Read the model definition and answer for the solid it produces. Units are mm, in the model's axes. A direction names the side the tool comes from. Give positions to 0.01 mm unless a question says otherwise; leave off trailing zeros. Order: outer loops, then holes, each group sorted by start corner. A loop starts at its lowest first (then second) coordinate and runs counter-clockwise, first axis right, second up. Notation, with made-up numbers: (49.25, -23.75) - (58.25, -23.75) arc R20 ccw to (58.25, -8.75) - close; hole circle Ø5 at (19, 63.25). An arc over 180 degrees is marked (long way). Write item = value, one per line.
```python
from build123d import *

# Parameters (mm, degrees)
F1_DEPTH = 5


with BuildPart() as f1:
    # F0 (on Front) → F1 (new body)
    with BuildSketch(Plane.XZ):
        Polygon((61.512955, -18.03444), (75.960928, 2.436688), (64.075245, 1.856776), (71.490157, 25.790645), (60.365404, 21.566239), (60.021432, 46.620035), (50.746576, 39.164648), (42.677391, 62.885931), (36.16032, 52.929348), (21.15579, 72.996113), (18.03444, 61.512955), (-2.436688, 75.960928), (-1.856776, 64.075245), (-25.790645, 71.490157), (-21.566239, 60.365404), (-46.620035, 60.021432), (-39.164648, 50.746576), (-62.885931, 42.677391), (-52.929348, 36.16032), (-72.996113, 21.15579), (-61.512955, 18.03444), (-75.960928, -2.436688), (-64.075245, -1.856776), (-71.490157, -25.790645), (-60.365404, -21.566239), (-60.021432, -46.620035), (-50.746576, -39.164648), (-42.677391, -62.885931), (-36.16032, -52.929348), (-21.15579, -72.996113), (-18.03444, -61.512955), (2.436688, -75.960928), (1.856776, -64.075245), (25.790645, -71.490157), (21.566239, -60.365404), (46.620035, -60.021432), (39.164648, -50.746576), (62.885931, -42.677391), (52.929348, -36.16032), (72.996113, -21.15579), align=None)
        with BuildLine():
            ThreePointArc((3.847568, 18.606349), (14.732681, 11.997837), (19, 0))
            ThreePointArc((19, 0), (-12.106443, -14.643566), (-3.572003, 18.661211))
            Line((-3.572003, 18.661211), (-3.572003, 23.642808))
            Line((-3.572003, 23.642808), (3.847568, 23.642808))
            Line((3.847568, 23.642808), (3.847568, 18.606349))
        make_face(mode=Mode.SUBTRACT)
    extrude(amount=F1_DEPTH)


solid = f1.part
```
1. Straight lines are drawn through the part: L1, parallel to Z at x = 56, y = -1.5; L2, parallel to Z at x = 16, y = -3.4; L3, parallel to X at y = -4.2, z = 5. For each, find the intervals that lie inside material, in ascending order. Write a range as [from, to].
Recorded:
L1 = [-45.02, -38.17], [-33.86, 43.39]
L2 = [-68.46, -10.25], [10.25, 62.95]
L3 = [-70.71, -18.33], [18.33, 65.05]
2. Flat-ended cylindrical pins translate along their axes: pin 1 (1 mm diameter, centred on x = 36.5, y = -4.5, fed in from +Z); pin 2 (2 mm diameter, centred on y = -3.5, z = -53.5, fed in from +X). Find the tip coordinate at first contact, or state that the pin passes through.
Recorded:
pin_1 = 54.21
pin_2 = 42.18
3. Section D-D (z = -30.5) is taken. Determine the outline of the cut face in (x, y).
Recorded:
outline = (-60.24, -5) - (60.5, -5) - (60.5, 0) - (-60.24, 0) - close
4. For faces 1 (the face through (28.763, -2.465, 62.822)), 2 (the face through (-28.763, -2.465, -62.822)), 3 (the face through (-62.822, -2.465, 28.763)), determine the directions among +Z, -Z, +X, -X, +Y, -Y from which every point of the face is accessible in a straight line to the end or side of a thin tool.
Recorded:
face_1 = +Z, +Y, -Y
face_2 = -Z, +Y, -Y
face_3 = -X, +Y, -Y
5. Section A-A (z = -13) is taken. Determine the outline of the cut face in (x, y).
Recorded:
outline = (-67.53, -5) - (-13.86, -5) - (-13.86, 0) - (-67.53, 0) - close; (13.86, -5) - (65.07, -5) - (65.07, 0) - (13.86, 0) - close
6. Determine the mould class of faces 4 (the face through (46.77, -2.46, 50.86)), 5 (the face through (-50.86, -2.46, 46.77)), 6 (the face through (-46.77, -2.46, -50.86)), 7 (the face through (-67.335, -2.465, 19.617)) for opening direction Z: +Z half, -Z half, draft (parallel to the pull), parting line (faces both ways), or undercut.
Recorded:
face_4 = +Z half
face_5 = undercut
face_6 = -Z half
face_7 = undercut
7. Section B-B (x = 0) is taken. Determine the outline of the cut face in (y, z).
Recorded:
outline = (-5, -74.24) - (0, -74.24) - (0, -19) - (-5, -19) - close; (-5, 23.64) - (0, 23.64) - (0, 74.24) - (-5, 74.24) - close
8. Section C-C (x = 31) is taken. Determine the outline of the cut face in (y, z), and give its area (3 significant figures).
Recorded:
outline = (-5, -60.24) - (0, -60.24) - (0, 59.83) - (-5, 59.83) - close
area = 600 mm^2
